The figure shows three views and two pictorial views of one solid part (mm, origin at its lowest corner). Answer the questions. A direction names the side the tool comes from. Round coordinates to 2 decimals unless told otherwise and drop trailing zeros. Order: outer loops, then holes, each group sorted by start corner. A loop starts at its lowest first (then second) coordinate and runs counter-clockwise, first axis right, second up. Notation, with made-up numbers: (32.5, -9) - (36.5, -9) arc R26 cw to (36.5, 23) - close; hole circle Ø1 at (36.5, 11.25). An arc over 180 degrees is marked (long way). Use CSV: the item, a comma, the result in double quotes.
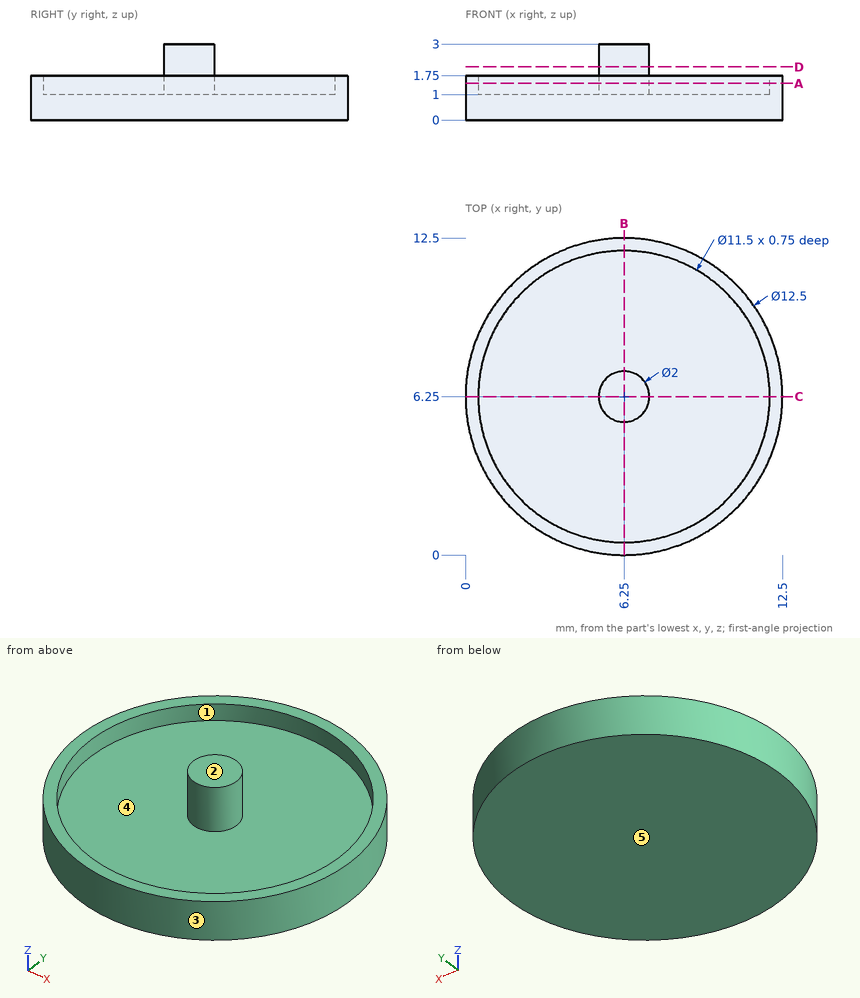
(1) Find the intervals of material crossed by L1, parallel to Y at x = 6.25, z = 1.4; L2, parallel to X at y = 5.5, z = 1.55; L3, parallel to Z at x = 6, y = 8.5, in increasing order. Write a range as from..to.
Findings below:
L1,"y = 0..0.5, 5.25..7.25, 12..12.5"
L2,"x = 0.05..0.55, 5.59..6.91, 11.95..12.45"
L3,"z = 0..1"
(2) Find section D-D (z = 2.1). Determine the outline of the cut face in (x, y), and give its area (3 significant figures).
Findings below:
outline,"circle Ø2 at (6.25, 6.25)"
area,"3.14 mm²"
(3) This flat-tipped pin is pushed along its axis until it touches: pin 1 (1.5 mm diameter, centred on x = 2.5, z = 0.5, fed in from -Y). Where does it stop, or does it pass through?
Findings below:
pin 1,"stops at y = 0.77"
(4) Find section A-A (z = 1.45). Determine the outline of the cut face in (x, y).
Findings below:
outline,"circle Ø12.5 at (6.25, 6.25); circle Ø2 at (6.25, 6.25); hole circle Ø11.5 at (6.25, 6.25)"
(5) For the marked faces 4 and 5, determine the directions among +Z, -Z, +X, -X, +Y, -Y from which every point of the face is accessible in a straight line to the end or side of a thin tool.
Findings below:
face 4,"+Z"
face 5,"-Z, +X, -X, +Y, -Y"
(6) The mould has two halves that part along Y. Classify the marked faces 1, 2 and 3: released by +Y, released by -Y, zero draft, split by the parting line, or undercut.
Findings below:
face 1,"undercut"
face 2,"zero draft"
face 3,"split by the parting line"
(7) Find section B-B (x = 6.25). Determine the outline of the cut face in (y, z), and give its area (4 significant figures).
Findings below:
outline,"(0, 0) - (12.5, 0) - (12.5, 1.75) - (12, 1.75) - (12, 1) - (7.25, 1) - (7.25, 3) - (5.25, 3) - (5.25, 1) - (0.5, 1) - (0.5, 1.75) - (0, 1.75) - close"
area,"17.25 mm²"
